Geometry check sheet. Reference: the model listing, model coordinates, mm. Face numbers are marked on the shaded views. A direction names the side the tool comes from. Round coordinates to 2 decimals unless told otherwise and drop trailing zeros. Loops run counter-clockwise (first coordinate to the right, second up) from the corner with the lowest first, then second, coordinate; pieces in that order, holes last. Notation, with made-up numbers: (56, 75.5) - (65, 75.5) arc R22 ccw to (65, 88.5) - close; hole circle Ø7 at (14.25, 0.5). An arc over 180 degrees is marked (long way). Answer as CSV lines item,"result". Start each with the question number.
1) Depth check by flat-ended pin: P1, Ø5, axis at y = -45.5, z = 49.5, coming from the +X side; P2, Ø2, axis at y = -73, z = 45, coming from the +X side; P3, Ø3, axis at y = -75, z = 35, coming from the +X side; P4, Ø10, axis at x = -56, y = -84, coming from the -Z side. Enter the tip coordinate at first touch or a pass-through.
2) Draft check along Y on the marked faces 6, 7 and 8. Enter one of: released by +Y, released by -Y, zero draft, split by the parting line, or undercut.
3) Cross-section at D-D on y = -73. Record the boundary of the cut face in (x, z), and give its area (3 significant figures).
4) Cross-section at A-A on y = -30. Record the boundary of the cut face in (x, z), and give its area (3 significant figures).
5) Access from +Z, -Z, +X, -X, +Y, -Y to the whole of each face (thin tool, end or side, straight path). Record for the marked faces 1, 2, 3, 4 and 5.
6) Cross-section at C-C on x = -34.5. Record the boundary of the cut face in (y, z), and give its area (3 significant figures).
7) Thickness scan on line 1 along Y through (x, z) = (-45, 22); line 2 along Y through (x, z) = (-34.5, 65.5); line 3 along X through (y, z) = (-76, 39). Record the ranges inside material, lowest first.
8) Cross-section at B-B on z = 22. Record the boundary of the cut face in (x, y), and give its area (3 significant figures).
from build123d import *

# Parameters (mm, degrees)
F0_R     = 28.604238
F1_DEPTH = 25.4
F3_DEPTH = 25.4
F5_DEPTH = 25.4
F6_R     = 6.17176
F7_DEPTH = 25.4


with BuildPart() as f1:
    # F0 (on Front) → F1 (new body)
    with BuildSketch(Plane.XZ):
        with Locations((-42.036779, 40.495433)):
            Circle(F0_R)
    extrude(amount=F1_DEPTH)

    # F2 (on face) → F3 (join)
    with BuildSketch(Plane.XZ.offset(25.4)):
        Polygon((-17.834256, 40.347526), (-29.807427, 61.381479), (-54.00995, 61.529386), (-66.239302, 40.643339), (-54.266131, 19.609387), (-30.063609, 19.46148), align=None)
    extrude(amount=F3_DEPTH)

    # F4 (on face) → F5 (join)
    with BuildSketch(Plane.XZ.offset(50.8)):
        Polygon((-29.067197, 40.669558), (-33.147233, 49.849639), (-42.173565, 54.259393), (-51.922672, 51.835446), (-57.832837, 43.71199), (-57.13863, 33.69008), (-50.164877, 26.45908), (-40.174675, 25.402454), (-31.84255, 31.01461), align=None)
    extrude(amount=F5_DEPTH)

    # F6 (on face) → F7 (join)
    with BuildSketch(Plane.XZ.offset(76.2)):
        with Locations((-44.278741, 38.533714)):
            Circle(F6_R)
    extrude(amount=F7_DEPTH)


solid = f1.part
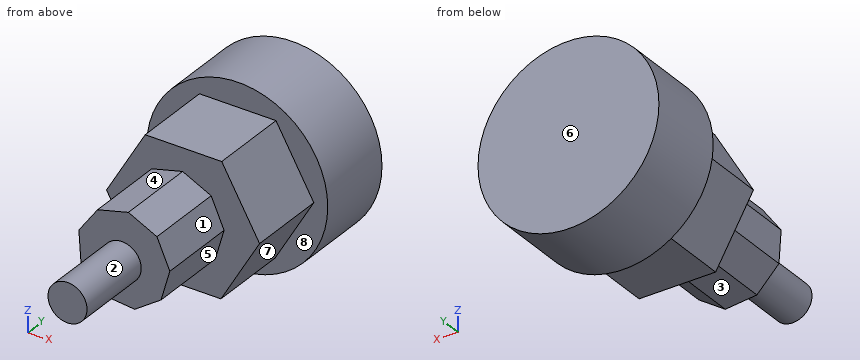
Answer block:
1,P1,"stops at x = -21.62"
1,P2,"stops at x = -30.55"
1,P3,"stops at x = -30.27"
1,P4,"passes through"
2,face 6,"released by +Y"
2,face 7,"zero draft"
2,face 8,"released by -Y"
3,outline,"(-57.83, 43.71) - (-57.14, 33.69) - (-50.16, 26.46) - (-40.17, 25.4) - (-31.84, 31.01) - (-29.07, 40.67) - (-33.15, 49.85) - (-42.17, 54.26) - (-51.92, 51.84) - close"
3,area,"624 mm^2"
4,outline,"(-66.24, 40.64) - (-54.27, 19.61) - (-30.06, 19.46) - (-17.83, 40.35) - (-29.81, 61.38) - (-54.01, 61.53) - close"
4,area,"1,520 mm^2"
5,face 1,"+Z, +X, -Y"
5,face 2,"-Y"
5,face 3,"-Z, -X, -Y"
5,face 4,"+Z, -X, -Y"
5,face 5,"-Z, +X, -Y"
6,outline,"(-76.2, 29.22) - (-50.8, 29.22) - (-50.8, 19.49) - (-25.4, 19.49) - (-25.4, 12.9) - (0, 12.9) - (0, 68.09) - (-25.4, 68.09) - (-25.4, 61.41) - (-50.8, 61.41) - (-50.8, 50.51) - (-76.2, 50.51) - close"
6,area,"3,010 mm^2"
7,line 1,"y = -50.8 to 0"
7,line 2,"y = -25.4 to 0"
7,line 3,"x = -57.51 to -29.55"
8,outline,"(-63.86, -25.4) - (-55.63, -25.4) - (-55.63, -50.8) - (-28.58, -50.8) - (-28.58, -25.4) - (-20.22, -25.4) - (-20.22, 0) - (-63.86, 0) - close"
8,area,"1,800 mm^2"
